Geometry: final body of the model. Coordinates: model frame, mm. Give positions to 0.01 mm unless a question says otherwise; leave off trailing zeros. Order: outer loops, then holes, each group sorted by start corner. A loop starts at its lowest first (then second) coordinate and runs counter-clockwise, first axis right, second up. Notation, with made-up numbers: (-33, 35.25) -> (0, 35.25) arc R30 ccw to (0, 65.25) -> close; hole circle Ø8 at (-23.75, 5.5). An arc over 180 degrees is marked (long way). Write item = value, one per line.
```python
from build123d import *

# Parameters (mm, degrees)
SKETCH_1_R          = 178
EXTRUDE_1_DEPTH     = 4
SKETCH_2_R          = 10
SKETCH_2_R_2        = 5.2
CUT_EXTRUDE_1_DEPTH = 10
SKETCH_4_R          = 54.5
CUT_EXTRUDE_2_DEPTH = 10
SKETCH_5_R          = 2
CUT_EXTRUDE_3_DEPTH = 10
CUT_EXTRUDE_4_DEPTH = 10
SKETCH_11_W         = 100
SKETCH_11_H         = 3
CUT_EXTRUDE_5_DEPTH = 10
SKETCH_13_R         = 15
CUT_EXTRUDE_6_DEPTH = 10


with BuildPart() as part:
    # 草图1 → 凸台-拉伸1 (new body)
    with BuildSketch(Plane(origin=(0, 0, 0), x_dir=(1, 0, 0), z_dir=(0, 1, 0))):
        Circle(SKETCH_1_R)
    extrude(amount=EXTRUDE_1_DEPTH)

    # 草图2 → 切除-拉伸1 (cut)
    with BuildSketch(Plane(origin=(0, 4, 0), x_dir=(1, 0, 0), z_dir=(0, 1, 0))):
        with Locations((115.258405333, 115.258405333)):
            Circle(SKETCH_2_R)
        with Locations((-90.216925784, -106.480381752)):
            Circle(SKETCH_2_R_2)
        with Locations((-106.480381752, -90.216925784)):
            Circle(SKETCH_2_R_2)
        with Locations((115.258405333, -115.258405333)):
            Circle(SKETCH_2_R)
        with Locations((-115.258405333, -115.258405333)):
            Circle(SKETCH_2_R)
        with Locations((-115.258405333, 115.258405333)):
            Circle(SKETCH_2_R)
        with Locations((-90.216925784, 106.480381752)):
            Circle(SKETCH_2_R_2)
        with Locations((-106.480381752, 90.216925784)):
            Circle(SKETCH_2_R_2)
        with Locations((106.480381752, 90.216925784)):
            Circle(SKETCH_2_R_2)
        with Locations((90.216925784, 106.480381752)):
            Circle(SKETCH_2_R_2)
        with Locations((90.216925784, -106.480381752)):
            Circle(SKETCH_2_R_2)
        with Locations((106.480381752, -90.216925784)):
            Circle(SKETCH_2_R_2)
    extrude(amount=-CUT_EXTRUDE_1_DEPTH, mode=Mode.SUBTRACT)

    # 草图4 → 切除-拉伸2 (cut)
    with BuildSketch(Plane.XZ):
        with Locations((80.5, 0)):
            Circle(SKETCH_4_R)
        with Locations((-80.5, 0)):
            Circle(SKETCH_4_R)
    extrude(amount=-CUT_EXTRUDE_2_DEPTH, mode=Mode.SUBTRACT)

    # 草图5 → 切除-拉伸3 (cut)
    with BuildSketch(Plane(origin=(0, 4, 0), x_dir=(1, 0, 0), z_dir=(0, 1, 0))):
        with Locations((-19.5, -14.8)):
            Circle(SKETCH_5_R)
        with Locations((-4.5, -14.8)):
            Circle(SKETCH_5_R)
        with Locations((-4.5, 14.8)):
            Circle(SKETCH_5_R)
        with Locations((-19.5, 14.8)):
            Circle(SKETCH_5_R)
        with Locations((4.5, -14.8)):
            Circle(SKETCH_5_R)
        with Locations((19.5, -14.8)):
            Circle(SKETCH_5_R)
        with Locations((19.5, 14.8)):
            Circle(SKETCH_5_R)
        with Locations((4.5, 14.8)):
            Circle(SKETCH_5_R)
        with Locations((-65.7, -61)):
            Circle(SKETCH_5_R)
        with Locations((-65.7, -76)):
            Circle(SKETCH_5_R)
        with Locations((-95.3, -61)):
            Circle(SKETCH_5_R)
        with Locations((-95.3, -76)):
            Circle(SKETCH_5_R)
        with Locations((-141.5, -14.8)):
            Circle(SKETCH_5_R)
        with Locations((-156.5, -14.8)):
            Circle(SKETCH_5_R)
        with Locations((-141.5, 14.8)):
            Circle(SKETCH_5_R)
        with Locations((-156.5, 14.8)):
            Circle(SKETCH_5_R)
        with Locations((-95.3, 61)):
            Circle(SKETCH_5_R)
        with Locations((-95.3, 76)):
            Circle(SKETCH_5_R)
        with Locations((-65.7, 61)):
            Circle(SKETCH_5_R)
        with Locations((-65.7, 76)):
            Circle(SKETCH_5_R)
        with Locations((95.3, 76)):
            Circle(SKETCH_5_R)
        with Locations((95.3, 61)):
            Circle(SKETCH_5_R)
        with Locations((65.7, 76)):
            Circle(SKETCH_5_R)
        with Locations((65.7, 61)):
            Circle(SKETCH_5_R)
        with Locations((156.5, -14.8)):
            Circle(SKETCH_5_R)
        with Locations((141.5, -14.8)):
            Circle(SKETCH_5_R)
        with Locations((156.5, 14.8)):
            Circle(SKETCH_5_R)
        with Locations((141.5, 14.8)):
            Circle(SKETCH_5_R)
        with Locations((65.7, -76)):
            Circle(SKETCH_5_R)
        with Locations((65.7, -61)):
            Circle(SKETCH_5_R)
        with Locations((95.3, -76)):
            Circle(SKETCH_5_R)
        with Locations((95.3, -61)):
            Circle(SKETCH_5_R)
    extrude(amount=-CUT_EXTRUDE_3_DEPTH, mode=Mode.SUBTRACT)

    # 草图8 → 切除-拉伸4 (cut)
    with BuildSketch(Plane.XZ):
        with BuildLine():
            Line((95.833188406, 150), (0, 150))
            Line((0, 150), (-95.833188406, 150))
            ThreePointArc((-95.833188406, 150), (0, 178), (95.833188406, 150))
        make_face()
        with BuildLine():
            Line((170, 52.763623833), (170, 0))
            Line((170, 0), (170, -52.763623833))
            ThreePointArc((170, -52.763623833), (178, 0), (170, 52.763623833))
        make_face()
        with BuildLine():
            Line((0, -150), (-95.833188406, -150))
            ThreePointArc((-95.833188406, -150), (0, -178), (95.833188406, -150))
            Line((95.833188406, -150), (0, -150))
        make_face()
        with BuildLine():
            Line((-170, 0), (-170, -52.763623833))
            ThreePointArc((-170, -52.763623833), (-178, 0), (-170, 52.763623833))
            Line((-170, 52.763623833), (-170, 0))
        make_face()
    extrude(amount=-CUT_EXTRUDE_4_DEPTH, mode=Mode.SUBTRACT)

    # 草图11 → 切除-拉伸5 (cut)
    with BuildSketch(Plane.XZ):
        with Locations((0, -86.5)):
            Rectangle(SKETCH_11_W, SKETCH_11_H)
        Polygon((65, -135), (30, -135), (30, -119), (30, -103), (65, -103), align=None)
        Polygon((-65, -119), (-65, -103), (-30, -103), (-30, -119), (-30, -135), (-65, -135), align=None)
        with Locations((0, 86.5)):
            Rectangle(SKETCH_11_W, SKETCH_11_H)
        Polygon((-65, 119), (-65, 103), (-30, 103), (-30, 119), (-30, 135), (-65, 135), align=None)
        Polygon((65, 103), (65, 135), (30, 135), (30, 119), (30, 103), align=None)
    extrude(amount=-CUT_EXTRUDE_5_DEPTH, mode=Mode.SUBTRACT)

    # 草图13 → 切除-拉伸6 (cut)
    with BuildSketch(Plane.XZ):
        with Locations((0, -50)):
            Circle(SKETCH_13_R)
        with Locations((0, 50)):
            Circle(SKETCH_13_R)
    extrude(amount=-CUT_EXTRUDE_6_DEPTH, mode=Mode.SUBTRACT)


solid = part.part
```
1) Mould query, pull axis X, two halves, no side actions, for faces 1 (the face through (113, 2, 125)), 2 (the face through (141, 1.97, 108.64)), 3 (the face through (-141, 1.97, -108.64)), 4 (the face through (-123.75, 1.97, -33.16)). Classes: +X half, -X half, draft (parallel to the pull), parting line (faces both ways), or undercut.
Check sheet entries:
face_1 = undercut
face_2 = +X half
face_3 = -X half
face_4 = undercut
2) First-contact query: P1, Ø1.5, axis at y = 3.5, z = -100, coming from the -X side; P2, Ø1, axis at y = 2.5, z = 118, coming from the -X side. Flat tips, straight axial feed; report the tip coordinate or a pass-through.
Check sheet entries:
P1 = -147.76
P2 = -133.71
3) Section query C-C (y = 2.9). Count the separate pieces of the cut face and the enclosed holes in it, plus the area to 3 significant figures.
Check sheet entries:
separate_pieces = 1
enclosed_holes = 54
area = 63,600 mm²
4) Section query B-B (x = -130). Output: boundary loops of the cut face in (y, z).
Check sheet entries:
outline = (0, -121.59) -> (4, -121.59) -> (4, -22.8) -> (0, -22.8) -> close; (0, 22.8) -> (4, 22.8) -> (4, 121.59) -> (0, 121.59) -> close
5) Line query: line 1 (Z direction, x = -0.5, y = 3.55); line 2 (Z direction, x = -103.5, y = 1.55); line 3 (X direction, y = 0.75, z = -2). Output: solid intervals per line, ascending. Write a range as from..to.
Check sheet entries:
line_1 = -150..-88, -85..-64.99, -35.01..35.01, 64.99..85, 88..150
line_2 = -144.82..-94.48, -85.96..-49.41, 49.41..85.96, 94.48..144.82
line_3 = -170..-134.96, -26.04..26.04, 134.96..170
6) Section query A-A (x = -80.5). Output: boundary loops of the cut face in (y, z), plus the area to 3 significant figures.
Check sheet entries:
outline = (0, -150) -> (4, -150) -> (4, -54.5) -> (0, -54.5) -> close; (0, 54.5) -> (4, 54.5) -> (4, 150) -> (0, 150) -> close
area = 764 mm²
